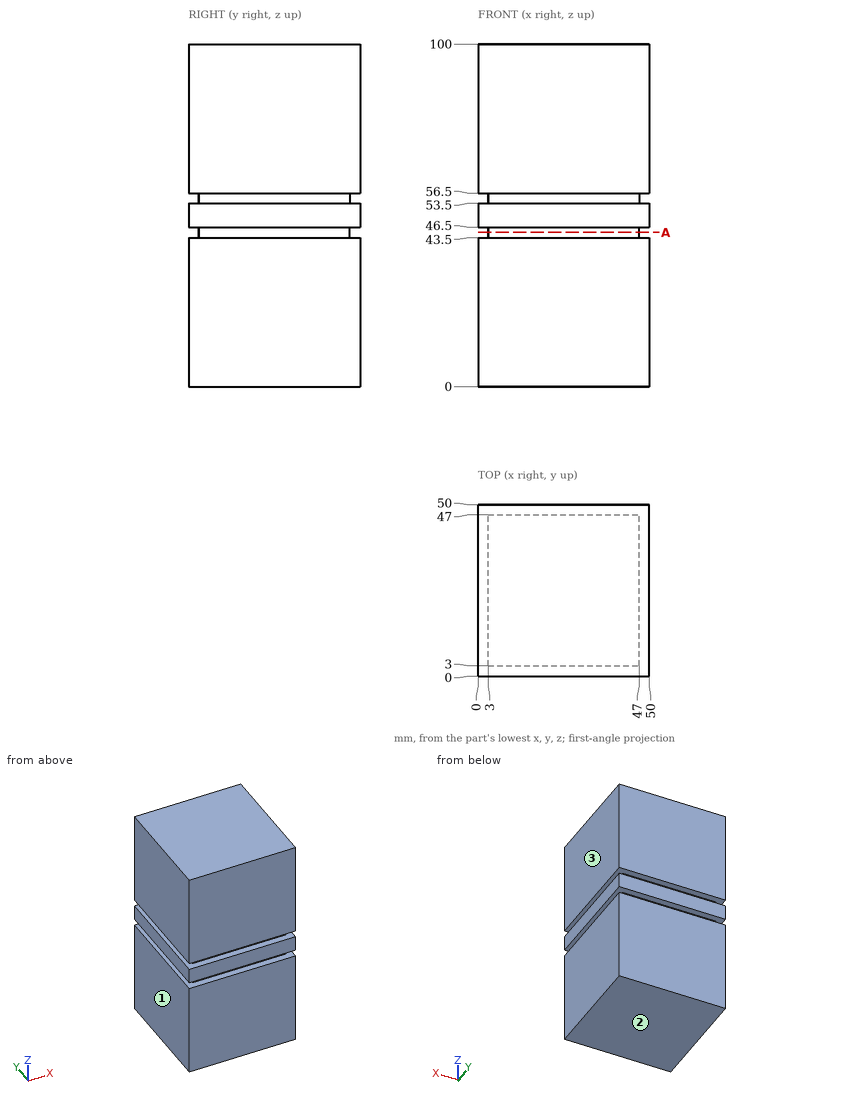
For this review, use the dimensioned drawing (mm, ordinates from the lowest corner) and the shaded views. Coordinates: 2 decimals unless noted, no trailing zeros. Write each loop counter-clockwise with the first axis right and the second up, starting at its lowest first coordinate (ties: lowest second). Pieces come first, ordered by that corner, then holes. Notation, with made-up numbers: (-16.5, -1.75) - (10.5, -1.75) arc R27 cw to (10.5, 34.25) - close; hole circle Ø1 at (-0.5, 16). An arc over 180 degrees is marked (long way). Answer in a Markdown table with one row per item. Add a question column.
Q1. Clearance check with flat-ended pins moving along their axes: pin 1 (25 mm diameter, centred on x = 26.5, y = 14.5, fed in from -Z); pin 2 (0.9 mm diameter, centred on x = 31, z = 45.5, fed in from +Y); pin 3 (2.5 mm diameter, centred on x = 19.5, z = 45, fed in from -Y); pin 4 (1.5 mm diameter, centred on y = 35, z = 55, fed in from +X). State where each tip first meets the part, or that it passes through.
Q2. To check wall thickness, follow line 1 along Y through (x, z) = (9, 55). State the ranges of the line that lie inside material, in increasing order. Write a range as from..to.
Q3. Draft analysis for pull direction X (two halves, no side actions). For the marked faces 1, 2 and 3, state which applies: +X half, -X half, draft (parallel to the pull), parting line (faces both ways), or undercut.
Q4. Consider section A-A on z = 45. Give the boundary of the cut face in (x, y), then the cut area to 3 significant figures.
Answers below:
| question | item | result |
|---|---|---|
| 1 | pin 1 | z = 0 |
| 1 | pin 2 | y = 47 |
| 1 | pin 3 | y = 3 |
| 1 | pin 4 | x = 47 |
| 2 | line 1 | 3..47 |
| 3 | face 1 | -X half |
| 3 | face 2 | draft |
| 3 | face 3 | +X half |
| 4 | outline | (3, 3) - (47, 3) - (47, 47) - (3, 47) - close |
| 4 | area | 1,940 mm² |
